```python
from build123d import *

# Parameters (mm, degrees)
BOSS_EXTRUDE1_DEPTH = 16
SKETCH2_W           = 1.78
SKETCH2_H           = 13.8
CUT_EXTRUDE3_DEPTH  = 17.538527746
SKETCH3_W           = 1.3
SKETCH3_H           = 13.8
CUT_EXTRUDE4_DEPTH  = 2.8
BOSS_EXTRUDE2_DEPTH = 3.4
SKETCH5_W           = 6.46
SKETCH5_H           = 15
BOSS_EXTRUDE3_DEPTH = 0.5
SKETCH7_W           = 1.78
SKETCH7_H           = 13.8
CUT_EXTRUDE5_DEPTH  = 17.718938363
SKETCH8_W           = 1.3
SKETCH8_H           = 13.8
CUT_EXTRUDE6_DEPTH  = 0.1
CUT_EXTRUDE7_START  = -1
CUT_EXTRUDE7_DEPTH  = 1
FILLET1_R           = 0.3
SKETCH10_W          = 7.46
SKETCH10_H          = 0.8
CUT_EXTRUDE9_DEPTH  = 17.718938363
SKETCH11_W          = 1.3
SKETCH11_H          = 0.4
BOSS_EXTRUDE4_DEPTH = 13.8


with BuildPart() as part:
    # Sketch1 → Boss-Extrude1 (new body)
    with BuildSketch(Plane.XY):
        Polygon((-3.73, 0), (3.73, 0), (3.73, 3.1), (2.43, 3.1), (2.43, 1.9), (0.65, 1.9), (0.65, 3.1), (-0.65, 3.1), (-0.65, 1.9), (-2.43, 1.9), (-2.43, 3.1), (-3.73, 3.1), align=None)
    extrude(amount=-BOSS_EXTRUDE1_DEPTH)

    # Sketch2 → Cut-Extrude3 (cut, through all)
    with BuildSketch(Plane(origin=(0, 1.9, 0), x_dir=(1, 0, 0), z_dir=(0, 1, 0))):
        with Locations((1.54, 8)):
            Rectangle(SKETCH2_W, SKETCH2_H)
    cut_extrude3 = extrude(amount=-CUT_EXTRUDE3_DEPTH, mode=Mode.SUBTRACT)

    # Mirror1: Cut-Extrude3 across plane
    add(cut_extrude3.mirror(Plane(origin=(0, 0, 0), x_dir=(0, 0, 1), z_dir=(1, 0, 0))), mode=Mode.SUBTRACT)

    # Sketch3 → Cut-Extrude4 (cut)
    with BuildSketch(Plane.XZ):
        with Locations((0, -8)):
            Rectangle(SKETCH3_W, SKETCH3_H)
    extrude(amount=-CUT_EXTRUDE4_DEPTH, mode=Mode.SUBTRACT)

    # Sketch4 → Boss-Extrude2 (add)
    with BuildSketch(Plane.XZ.offset(-2.8)):
        with BuildLine():
            Line((0.65, -7.15), (0.65, -8.65))
            ThreePointArc((0.65, -8.65), (0, -9.3), (-0.65, -8.65))
            Line((-0.65, -8.65), (-0.65, -7.15))
            ThreePointArc((-0.65, -7.15), (0, -6.5), (0.65, -7.15))
        make_face()
    extrude(amount=BOSS_EXTRUDE2_DEPTH)

    # Sketch5 → Boss-Extrude3 (add)
    with BuildSketch(Plane.XZ):
        with Locations((0, -8)):
            Rectangle(SKETCH5_W, SKETCH5_H)
    extrude(amount=BOSS_EXTRUDE3_DEPTH)

    # Sketch7 → Cut-Extrude5 (cut, through all)
    with BuildSketch(Plane(origin=(0, 0, 0), x_dir=(1, 0, 0), z_dir=(0, 1, 0))):
        with Locations((-1.54, 8)):
            Rectangle(SKETCH7_W, SKETCH7_H)
    cut_extrude5 = extrude(amount=-CUT_EXTRUDE5_DEPTH, mode=Mode.SUBTRACT)

    # Mirror2: Cut-Extrude5 across plane
    add(cut_extrude5.mirror(Plane(origin=(0, 0, 0), x_dir=(0, 0, 1), z_dir=(1, 0, 0))), mode=Mode.SUBTRACT)

    # Sketch8 → Cut-Extrude6 (cut)
    with BuildSketch(Plane.XZ.offset(0.5)):
        with Locations((0, -8)):
            Rectangle(SKETCH8_W, SKETCH8_H)
    extrude(amount=CUT_EXTRUDE6_DEPTH, mode=Mode.SUBTRACT)

    # Sketch9 → Cut-Extrude7 (cut)
    with BuildSketch(Plane.XZ.offset(0.5).offset(CUT_EXTRUDE7_START)):
        with BuildLine():
            Line((-0.65, -14.9), (0.65, -14.9))
            Line((0.65, -14.9), (0.65, -8.65))
            ThreePointArc((0.65, -8.65), (0, -9.3), (-0.65, -8.65))
            Line((-0.65, -8.65), (-0.65, -14.9))
        make_face()
    cut_extrude7 = extrude(amount=CUT_EXTRUDE7_DEPTH, mode=Mode.SUBTRACT)

    # Mirror3: Cut-Extrude7 across plane
    add(cut_extrude7.mirror(Plane.XY.offset(-7.9)), mode=Mode.SUBTRACT)

    # Fillet1
    fillet1_edges = [part.edges().sort_by_distance(p)[0] for p in [
        (3.23, -0.25, -0.5),
        (-3.23, -0.25, -0.5),
        (-3.23, -0.25, -15.5),
        (3.23, -0.25, -15.5),
    ]]
    fillet(fillet1_edges, radius=FILLET1_R)

    # Sketch10 → Cut-Extrude9 (cut, through all)
    with BuildSketch(Plane.XY):
        with Locations((0, 2.7)):
            Rectangle(SKETCH10_W, SKETCH10_H)
    extrude(amount=-CUT_EXTRUDE9_DEPTH, mode=Mode.SUBTRACT)


with BuildPart() as cut_extrude9_piece_1:
    # of the separate pieces the step leaves, piece 1, a body of its own (cut_extrude9_pieces)
    add(part.part.solids().sort_by_distance((-2.93, 0, -0.5))[0])



with BuildPart() as cut_extrude9_piece_2:
    # of the separate pieces the step leaves, piece 2, a body of its own (cut_extrude9_pieces)
    add(part.part.solids().sort_by_distance((-0.65, -0.5, -7.15))[0])


with BuildPart() as cut_extrude9_piece_1_1:
    add(cut_extrude9_piece_1.part)

    add(cut_extrude9_piece_2.part)  # Boss-Extrude4 merges Cut-Extrude9 piece 2
    # Sketch11 → Boss-Extrude4 (add)
    with BuildSketch(Plane(origin=(0, 0, -1.1), x_dir=(-1, 0, 0), z_dir=(0, 0, -1))):
        with Locations((0, 2.1)):
            Rectangle(SKETCH11_W, SKETCH11_H)
    extrude(amount=BOSS_EXTRUDE4_DEPTH)


solid = cut_extrude9_piece_1_1.part
```
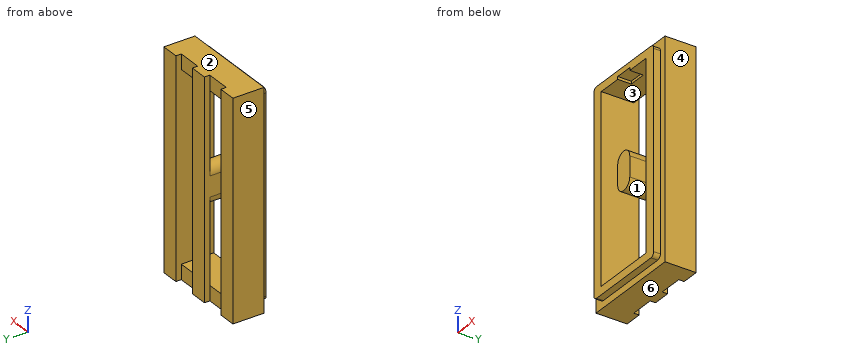
Geometry check sheet. Reference: the model listing, model coordinates, mm. Face numbers are marked on the shaded views. A direction names the side the tool comes from. Give positions to 0.01 mm unless a question says otherwise; leave off trailing zeros. Loops run counter-clockwise (first coordinate to the right, second up) from the corner with the lowest first, then second, coordinate; pieces in that order, holes last. Notation, with made-up numbers: M 51,-16.75 L 89,-16.75 A17 cw 89,3.25 Z; hole C -10.75,-19.5 d11. An arc over 180 degrees is marked long. Answer as CSV lines item,"result".
Item 1: Depth check by flat-ended pin: P1, Ø0.9, axis at x = -1.5, z = -0.5, coming from the +Y side. Enter the tip coordinate at first touch or a pass-through.
Values:
P1,"stops at y = 1.9"
Item 2: Material ranges on line 1 (X direction, y = 2.1, z = -2.25); line 2 (X direction, y = 1.1, z = -10.75); line 3 (X direction, y = -0.25, z = -9.75), recorded low to high.
Values:
line 1,"x = -3.73 to -2.43, -0.65 to 0.65, 2.43 to 3.73"
line 2,"x = -3.73 to -2.43, 2.43 to 3.73"
line 3,"x = -3.23 to -2.43, 2.43 to 3.23"
Item 3: Release check for a two-part mould opening along X. For the marked faces 3, 4, 5 and 6 record: pulls with the +X half, pulls with the -X half, needs draft (parallel to the pull), parting line crosses it, or undercut.
Values:
face 3,"undercut"
face 4,"pulls with the +X half"
face 5,"pulls with the -X half"
face 6,"needs draft"
Item 4: Access from +Z, -Z, +X, -X, +Y, -Y to the whole of each face (thin tool, end or side, straight path). Record for the marked faces 1 and 2.
Values:
face 1,"-Y"
face 2,"+Z, +X, -X, +Y, -Y"
Item 5: Cross-section at D-D on x = 2.25. Record the cut outline in (y, z), and give its area (3 significant figures).
Values:
outline,"M -0.5,-15.5 L 0,-15.5 L 0,-16 L 1.9,-16 L 1.9,-14.9 L -0.5,-14.9 Z; M -0.5,-1.1 L 1.9,-1.1 L 1.9,0 L 0,0 L 0,-0.5 L -0.5,-0.5 Z"
area,"4.78 mm²"
Item 6: Cross-section at C-C on y = -0.25. Record the cut outline in (x, z).
Values:
outline,"M -3.23,-15.2 A0.3 ccw -2.93,-15.5 L 2.93,-15.5 A0.3 ccw 3.23,-15.2 L 3.23,-0.8 A0.3 ccw 2.93,-0.5 L -2.93,-0.5 A0.3 ccw -3.23,-0.8 Z; M -0.65,-8.65 A0.65 ccw 0.65,-8.65 L 0.65,-7.15 A0.65 ccw -0.65,-7.15 Z; hole M -2.43,-14.9 L 2.43,-14.9 L 2.43,-1.1 L 0.65,-1.1 L 0.65,-0.9 L -0.65,-0.9 L -0.65,-1.1 L -2.43,-1.1 Z"
Item 7: Cross-section at B-B on z = -4.75. Record the cut outline in (x, y), and give its area (3 significant figures).
Values:
outline,"M -3.73,0 L -3.23,0 L -3.23,-0.5 L -2.43,-0.5 L -2.43,2.3 L -3.73,2.3 Z; M -0.65,1.9 L 0.65,1.9 L 0.65,2.3 L -0.65,2.3 Z; M 2.43,-0.5 L 3.23,-0.5 L 3.23,0 L 3.73,0 L 3.73,2.3 L 2.43,2.3 Z"
area,"7.30 mm²"
Item 8: Cross-section at A-A on y = 2.05. Record the cut outline in (x, z).
Values:
outline,"M -3.73,-16 L -2.43,-16 L -2.43,0 L -3.73,0 Z; M -0.65,-16 L 0.65,-16 L 0.65,0 L -0.65,0 Z; M 2.43,-16 L 3.73,-16 L 3.73,0 L 2.43,0 Z"
